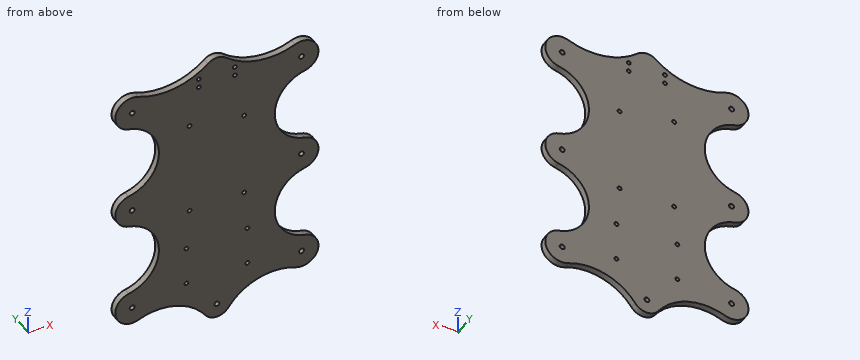
```python
from build123d import *

# Parameters (mm, degrees)
BOSS_EXTRUDE1_DEPTH = 6
SKETCH2_R           = 2.2
CUT_EXTRUDE1_DEPTH  = 235.538376391
CUT_EXTRUDE2_REACH  = 236.538
SKETCH3_R           = 1.7
CUT_EXTRUDE4_REACH  = 236.538
SKETCH5_R           = 2.2
CUT_EXTRUDE5_REACH  = 236.538
SKETCH6_R           = 1.7
SKETCH6_R_2         = 1.75
CUT_EXTRUDE6_REACH  = 236.538
SKETCH7_R           = 1.75


with BuildPart() as part:
    # Sketch1 → Boss-Extrude1 (new body)
    with BuildSketch(Plane(origin=(0, 0, 0), x_dir=(1, 0, 0), z_dir=(0, 1, 0))):
        with BuildLine():
            ThreePointArc((-69.425886336, 13.925848515), (-89.364705834, 4.31916963), (-78.030296498, -14.690721668))
            ThreePointArc((-78.030296498, -14.690721668), (-51.297958971, -47.499999875), (-78.030296252, -80.309278281))
            ThreePointArc((-78.030296252, -80.309278281), (-90, -94.999999814), (-78.030296616, -109.690721644))
            ThreePointArc((-78.030296616, -109.690721644), (-51.297958971, -142.5), (-78.030296616, -175.309278356))
            ThreePointArc((-78.030296616, -175.309278356), (-89.351304792, -194.363490663), (-69.340019232, -203.891170494))
            ThreePointArc((-69.340019232, -203.891170494), (-37.34886135, -200.189043247), (-8.051740928, -213.561352835))
            ThreePointArc((-8.051740928, -213.561352835), (-6.73e-07, -216.5), (8.051739898, -213.561353702))
            ThreePointArc((8.051739898, -213.561353702), (37.348860289, -200.189043415), (69.340018489, -203.891170192))
            ThreePointArc((69.340018489, -203.891170192), (89.351304588, -194.363491335), (78.030297206, -175.309278478))
            ThreePointArc((78.030297206, -175.309278478), (51.297958971, -142.500000301), (78.030296616, -109.690721644))
            ThreePointArc((78.030296616, -109.690721644), (90, -95.000000257), (78.03029712, -80.30927846))
            ThreePointArc((78.03029712, -80.30927846), (51.297958971, -47.500000257), (78.030296616, -14.690721644))
            ThreePointArc((78.030296616, -14.690721644), (89.364705852, 4.319169572), (69.425886562, 13.925848605))
            ThreePointArc((69.425886562, 13.925848605), (36.800743446, 12.358424364), (10.169102241, 31.26906869))
            ThreePointArc((10.169102241, 31.26906869), (2.26e-07, 36.5), (-10.169101978, 31.269069058))
            ThreePointArc((-10.169101978, 31.269069058), (-36.800743112, 12.358424462), (-69.425886336, 13.925848515))
        make_face()
    extrude(amount=BOSS_EXTRUDE1_DEPTH)

    # Sketch2 → Cut-Extrude1 (cut, through all)
    with BuildSketch(Plane.XZ):
        with Locations(Location((-75, 190, 0), (0, 0, 270))):
            Circle(SKETCH2_R)
        with Locations(Location((-75, 95, 0), (0, 0, 270))):
            Circle(SKETCH2_R)
        with Locations(Location((-75, 0, 0), (0, 0, 270))):
            Circle(SKETCH2_R)
        with Locations(Location((75, 0, 0), (0, 0, 270))):
            Circle(SKETCH2_R)
        with Locations(Location((75, 95, 0), (0, 0, 270))):
            Circle(SKETCH2_R)
        with Locations(Location((75, 190, 0), (0, 0, 270))):
            Circle(SKETCH2_R)
    extrude(amount=-CUT_EXTRUDE1_DEPTH, mode=Mode.SUBTRACT)

    # Sketch3 → Cut-Extrude2 (cut, up to next)
    with BuildSketch(Plane(origin=(0, 6, 0), x_dir=(1, 0, 0), z_dir=(0, 1, 0)), mode=Mode.PRIVATE) as cut_extrude2_sk1:
        with Locations(Location((-16, -193.5, 0), (0, 0, 270))):
            Circle(SKETCH3_R)
    cut_extrude2_tool1 = extrude(cut_extrude2_sk1.sketch, amount=-CUT_EXTRUDE2_REACH, mode=Mode.PRIVATE) & part.part
    # Sketch3 → Cut-Extrude2 (cut, up to next)
    with BuildSketch(Plane(origin=(0, 6, 0), x_dir=(1, 0, 0), z_dir=(0, 1, 0)), mode=Mode.PRIVATE) as cut_extrude2_sk2:
        with Locations(Location((16, -193.5, 0), (0, 0, 270))):
            Circle(SKETCH3_R)
    cut_extrude2_tool2 = extrude(cut_extrude2_sk2.sketch, amount=-CUT_EXTRUDE2_REACH, mode=Mode.PRIVATE) & part.part
    # Sketch3 → Cut-Extrude2 (cut, up to next)
    with BuildSketch(Plane(origin=(0, 6, 0), x_dir=(1, 0, 0), z_dir=(0, 1, 0)), mode=Mode.PRIVATE) as cut_extrude2_sk3:
        with Locations(Location((-16, -201.5, 0), (0, 0, 270))):
            Circle(SKETCH3_R)
    cut_extrude2_tool3 = extrude(cut_extrude2_sk3.sketch, amount=-CUT_EXTRUDE2_REACH, mode=Mode.PRIVATE) & part.part
    # Sketch3 → Cut-Extrude2 (cut, up to next)
    with BuildSketch(Plane(origin=(0, 6, 0), x_dir=(1, 0, 0), z_dir=(0, 1, 0)), mode=Mode.PRIVATE) as cut_extrude2_sk4:
        with Locations(Location((16, -201.5, 0), (0, 0, 270))):
            Circle(SKETCH3_R)
    cut_extrude2_tool4 = extrude(cut_extrude2_sk4.sketch, amount=-CUT_EXTRUDE2_REACH, mode=Mode.PRIVATE) & part.part
    add(cut_extrude2_tool1.solids().sort_by_distance((-16, 6, 193.5))[0], mode=Mode.SUBTRACT)
    add(cut_extrude2_tool2.solids().sort_by_distance((16, 6, 193.5))[0], mode=Mode.SUBTRACT)
    add(cut_extrude2_tool3.solids().sort_by_distance((-16, 6, 201.5))[0], mode=Mode.SUBTRACT)
    add(cut_extrude2_tool4.solids().sort_by_distance((16, 6, 201.5))[0], mode=Mode.SUBTRACT)

    # Sketch5 → Cut-Extrude4 (cut, up to next)
    with BuildSketch(Plane(origin=(0, 6, 0), x_dir=(1, 0, 0), z_dir=(0, 1, 0)), mode=Mode.PRIVATE) as cut_extrude4_sk1:
        with Locations(Location((0, 24, 0), (0, 0, 270))):
            Circle(SKETCH5_R)
    cut_extrude4_tool1 = extrude(cut_extrude4_sk1.sketch, amount=-CUT_EXTRUDE4_REACH, mode=Mode.PRIVATE) & part.part
    add(cut_extrude4_tool1.solids().sort_by_distance((0, 6, -24))[0], mode=Mode.SUBTRACT)

    # Sketch6 → Cut-Extrude5 (cut, up to next)
    with BuildSketch(Plane(origin=(0, 6, 0), x_dir=(1, 0, 0), z_dir=(0, 1, 0)), mode=Mode.PRIVATE) as cut_extrude5_sk1:
        with Locations(Location((-27, -6, 0), (0, 0, 270))):
            Circle(SKETCH6_R)
    cut_extrude5_tool1 = extrude(cut_extrude5_sk1.sketch, amount=-CUT_EXTRUDE5_REACH, mode=Mode.PRIVATE) & part.part
    # Sketch6 → Cut-Extrude5 (cut, up to next)
    with BuildSketch(Plane(origin=(0, 6, 0), x_dir=(1, 0, 0), z_dir=(0, 1, 0)), mode=Mode.PRIVATE) as cut_extrude5_sk2:
        with Locations(Location((27, -6, 0), (0, 0, 270))):
            Circle(SKETCH6_R_2)
    cut_extrude5_tool2 = extrude(cut_extrude5_sk2.sketch, amount=-CUT_EXTRUDE5_REACH, mode=Mode.PRIVATE) & part.part
    # Sketch6 → Cut-Extrude5 (cut, up to next)
    with BuildSketch(Plane(origin=(0, 6, 0), x_dir=(1, 0, 0), z_dir=(0, 1, 0)), mode=Mode.PRIVATE) as cut_extrude5_sk3:
        with Locations(Location((-27, -40, 0), (0, 0, 270))):
            Circle(SKETCH6_R)
    cut_extrude5_tool3 = extrude(cut_extrude5_sk3.sketch, amount=-CUT_EXTRUDE5_REACH, mode=Mode.PRIVATE) & part.part
    # Sketch6 → Cut-Extrude5 (cut, up to next)
    with BuildSketch(Plane(origin=(0, 6, 0), x_dir=(1, 0, 0), z_dir=(0, 1, 0)), mode=Mode.PRIVATE) as cut_extrude5_sk4:
        with Locations(Location((27, -40, 0), (0, 0, 270))):
            Circle(SKETCH6_R_2)
    cut_extrude5_tool4 = extrude(cut_extrude5_sk4.sketch, amount=-CUT_EXTRUDE5_REACH, mode=Mode.PRIVATE) & part.part
    add(cut_extrude5_tool1.solids().sort_by_distance((-27, 6, 6))[0], mode=Mode.SUBTRACT)
    add(cut_extrude5_tool2.solids().sort_by_distance((27, 6, 6))[0], mode=Mode.SUBTRACT)
    add(cut_extrude5_tool3.solids().sort_by_distance((-27, 6, 40))[0], mode=Mode.SUBTRACT)
    add(cut_extrude5_tool4.solids().sort_by_distance((27, 6, 40))[0], mode=Mode.SUBTRACT)

    # Sketch7 → Cut-Extrude6 (cut, up to next)
    with BuildSketch(Plane(origin=(0, 6, 0), x_dir=(1, 0, 0), z_dir=(0, 1, 0)), mode=Mode.PRIVATE) as cut_extrude6_sk1:
        with Locations(Location((-24.17, -76, 0), (0, 0, 270))):
            Circle(SKETCH7_R)
    cut_extrude6_tool1 = extrude(cut_extrude6_sk1.sketch, amount=-CUT_EXTRUDE6_REACH, mode=Mode.PRIVATE) & part.part
    # Sketch7 → Cut-Extrude6 (cut, up to next)
    with BuildSketch(Plane(origin=(0, 6, 0), x_dir=(1, 0, 0), z_dir=(0, 1, 0)), mode=Mode.PRIVATE) as cut_extrude6_sk2:
        with Locations(Location((24.17, -76, 0), (0, 0, 270))):
            Circle(SKETCH7_R)
    cut_extrude6_tool2 = extrude(cut_extrude6_sk2.sketch, amount=-CUT_EXTRUDE6_REACH, mode=Mode.PRIVATE) & part.part
    # Sketch7 → Cut-Extrude6 (cut, up to next)
    with BuildSketch(Plane(origin=(0, 6, 0), x_dir=(1, 0, 0), z_dir=(0, 1, 0)), mode=Mode.PRIVATE) as cut_extrude6_sk3:
        with Locations(Location((-24.17, -158.63, 0), (0, 0, 270))):
            Circle(SKETCH7_R)
    cut_extrude6_tool3 = extrude(cut_extrude6_sk3.sketch, amount=-CUT_EXTRUDE6_REACH, mode=Mode.PRIVATE) & part.part
    # Sketch7 → Cut-Extrude6 (cut, up to next)
    with BuildSketch(Plane(origin=(0, 6, 0), x_dir=(1, 0, 0), z_dir=(0, 1, 0)), mode=Mode.PRIVATE) as cut_extrude6_sk4:
        with Locations(Location((24.17, -151.13, 0), (0, 0, 270))):
            Circle(SKETCH7_R)
    cut_extrude6_tool4 = extrude(cut_extrude6_sk4.sketch, amount=-CUT_EXTRUDE6_REACH, mode=Mode.PRIVATE) & part.part
    add(cut_extrude6_tool1.solids().sort_by_distance((-24.17, 6, 76))[0], mode=Mode.SUBTRACT)
    add(cut_extrude6_tool2.solids().sort_by_distance((24.17, 6, 76))[0], mode=Mode.SUBTRACT)
    add(cut_extrude6_tool3.solids().sort_by_distance((-24.17, 6, 158.63))[0], mode=Mode.SUBTRACT)
    add(cut_extrude6_tool4.solids().sort_by_distance((24.17, 6, 151.13))[0], mode=Mode.SUBTRACT)


solid = part.part
```
Part model, mm, in its own coordinate system. Round coordinates to 2 decimals unless told otherwise and drop trailing zeros. Write each loop counter-clockwise with the first axis right and the second up, starting at its lowest first coordinate (ties: lowest second). Pieces come first, ordered by that corner, then holes. Notation, with made-up numbers: (-29.75, 81) -> (-8.75, 81) arc R37 ccw to (-8.75, 119) -> close; hole circle Ø4 at (-11, 35). An arc over 180 degrees is marked (long way). Return JSON: item names as keys, results as strings. Group by question number.
Q1. Pin check, flat tips, straight feed: pin 1 (1.5 mm diameter, centred on y = 2.5, z = 90.5, fed in from -X); pin 2 (2 mm diameter, centred on y = 4, z = 88, fed in from -X); pin 3 (1 mm diameter, centred on x = 53, y = 5.5, fed in from +Z). Stop position of each tip, or through.
Q2. Probe L1, parallel to Z at x = -15, y = 5.6; L2, parallel to Z at x = -27.5, y = 0.95; L3, parallel to X at y = 4.2, z = 6. List the from-to ranges inside material, lowest first. Write a range as [from, to].
Q3. Saw through at B-B on y = 3. State how many separate pieces and enclosed holes the cut face has, plus the area to 3 significant figures.
Q4. Saw through at A-A on x = 63. Write the cut outline in (y, z).
Q5. Saw through at C-C on z = 129. Write the cut outline in (x, y), plus the area to 3 significant figures.
Q6. Saw through at D-D on z = 183.5. Write the cut outline in (x, y), plus the area to 3 significant figures.
Answer:
{
 "1": {"pin 1": "x = -89.52", "pin 2": "x = -88.75", "pin 3": "z = 199.84"},
 "2": {"L1": "[-25.49, 192.13], [194.87, 200.13], [202.87, 208.51]", "L2": "[-16.13, 4.38], [7.62, 38.38], [41.62, 202.61]", "L3": "[-88.75, -28.7], [-25.3, 25.25], [28.75, 88.75]"},
 "3": {"separate pieces": "1", "enclosed holes": "19", "area": "30,700 mm2"},
 "4": {"outline": "(0, -11.85) -> (6, -11.85) -> (6, 22.06) -> (0, 22.06) -> close; (0, 72.94) -> (6, 72.94) -> (6, 117.06) -> (0, 117.06) -> close; (0, 167.94) -> (6, 167.94) -> (6, 201.71) -> (0, 201.71) -> close"},
 "5": {"outline": "(-54.14, 0) -> (54.14, 0) -> (54.14, 6) -> (-54.14, 6) -> close", "area": "650 mm2"},
 "6": {"outline": "(-88.52, 0) -> (88.52, 0) -> (88.52, 6) -> (-88.52, 6) -> close", "area": "1,060 mm2"}
}
